The model under review builds one solid part; all positions refer to its coordinate system, in mm. A direction names the side the tool comes from. Round coordinates to 2 decimals unless told otherwise and drop trailing zeros. Loops run counter-clockwise (first coordinate to the right, second up) from the corner with the lowest first, then second, coordinate; pieces in that order, holes last. Notation, with made-up numbers: (-25, 35.5) -> (-6, 35.5) arc R26 cw to (-6, 69.5) -> close; hole circle Ø2 at (-7.75, -30). An arc over 180 degrees is marked (long way). Use CSV: the item, a comma, the result in double quotes. Start each with the question number.
```python
from build123d import *

# Parameters (mm, degrees)
F0_W     = 64
F0_H     = 42
F1_DEPTH = 10
F2_W     = 60
F2_H     = 38
F3_DEPTH = 8
F4_W     = 10
F4_H     = 38
F5_DEPTH = 3
F6_W     = 4
F6_H     = 18
F7_DEPTH = 4


with BuildPart() as f1:
    # F0 (on Top) → F1 (new body)
    with BuildSketch(Plane.XY):
        with Locations((-36.174386, 25.71162)):
            Rectangle(F0_W, F0_H)
    extrude(amount=F1_DEPTH)

    # F2 (on face) → F3 (cut)
    with BuildSketch(Plane.XY.offset(10)):
        with Locations((-36.174389, 25.579226)):
            Rectangle(F2_W, F2_H)
    extrude(amount=-F3_DEPTH, mode=Mode.SUBTRACT)

    # F4 (on face) → F5 (join)
    with BuildSketch(Plane.XY.offset(2)):
        with Locations((-36.658923, 25.579226)):
            Rectangle(F4_W, F4_H)
    extrude(amount=F5_DEPTH)

    # F6 (on face) → F7 (join)
    with BuildSketch(Plane.XY.offset(5)):
        with Locations((-39.658923, 24.941399)):
            Rectangle(F6_W, F6_H)
    extrude(amount=F7_DEPTH)


solid = f1.part
```
1. For faces 1 (the face through (-40, 15.941, 7)), 2 (the face through (-4.174, 25, 5)), list the 3-axis set-ups (+Z, -Z, +X, -X, +Y, -Y) from which the entire face can be reached by the end or side of a thin tool; tool diameter is ignored.
2. Take a section at C-C, the plane y = 43. Give the boundary of the cut face in (x, z), then the cut area to 3 significant figures.
3. Take a section at B-B, the plane x = -55. Give the boundary of the cut face in (y, z).
4. Take a section at A-A, the plane z = 7.5. Give the boundary of the cut face in (x, y).
5. For line 1 along Y through (x, z) = (-38, 8.75); line 2 along X through (y, z) = (29.5, 6); line 3 along X through (y, z) = (29, 2.5), list the stretches that pass through material, from the lowest coordinate up. Write a range as from..to.
6. Take a section at D-D, the plane x = -41. Give the boundary of the cut face in (y, z).
7. Clearance check with flat-ended pins moving along their axes: P1, Ø10, axis at x = -10.5, y = 35, coming from the -Z side; P2, Ø3, axis at x = -37.5, y = 16, coming from the +Z side; P3, Ø7.5, axis at x = -58.5, y = 33.5, coming from the +Z side. State where each tip first meets the part, or that it passes through.
8. The part is to be moulded in two halves that separate along X. For faces 3 (the face through (-36, 26, 5)), 4 (the face through (-37, 46.712, 5)), 5 (the face through (-68.174, 25, 5)), say which applies: pulls with the +X half, pulls with the -X half, needs draft (parallel to the pull), parting line crosses it, or undercut.
Results:
1,face 1,"+Z"
1,face 2,"+Z, -Z, +X, +Y, -Y"
2,outline,"(-68.17, 0) -> (-4.17, 0) -> (-4.17, 10) -> (-6.17, 10) -> (-6.17, 2) -> (-31.66, 2) -> (-31.66, 5) -> (-41.66, 5) -> (-41.66, 2) -> (-66.17, 2) -> (-66.17, 10) -> (-68.17, 10) -> close"
2,area,"190 mm²"
3,outline,"(4.71, 0) -> (46.71, 0) -> (46.71, 10) -> (44.58, 10) -> (44.58, 2) -> (6.58, 2) -> (6.58, 10) -> (4.71, 10) -> close"
4,outline,"(-68.17, 4.71) -> (-4.17, 4.71) -> (-4.17, 46.71) -> (-68.17, 46.71) -> close; (-41.66, 15.94) -> (-37.66, 15.94) -> (-37.66, 33.94) -> (-41.66, 33.94) -> close; hole (-66.17, 6.58) -> (-6.17, 6.58) -> (-6.17, 44.58) -> (-66.17, 44.58) -> close"
5,line 1,"4.71..6.58, 15.94..33.94, 44.58..46.71"
5,line 2,"-68.17..-66.17, -41.66..-37.66, -6.17..-4.17"
5,line 3,"-68.17..-66.17, -41.66..-31.66, -6.17..-4.17"
6,outline,"(4.71, 0) -> (46.71, 0) -> (46.71, 10) -> (44.58, 10) -> (44.58, 5) -> (33.94, 5) -> (33.94, 9) -> (15.94, 9) -> (15.94, 5) -> (6.58, 5) -> (6.58, 10) -> (4.71, 10) -> close"
7,P1,"z = 0"
7,P2,"z = 9"
7,P3,"z = 2"
8,face 3,"undercut"
8,face 4,"needs draft"
8,face 5,"pulls with the -X half"
